Model file for the job. Use its own axes, mm. A direction names the side the tool comes from. Round coordinates to 2 decimals unless told otherwise and drop trailing zeros. Loops run counter-clockwise (first coordinate to the right, second up) from the corner with the lowest first, then second, coordinate; pieces in that order, holes last. Notation, with made-up numbers: (44.5, 82) - (58.5, 82) arc R32 ccw to (58.5, 118) - close; hole circle Ø1 at (-20, 22). An arc over 180 degrees is marked (long way). Use one line per item in the form item = value.
Autodesk Inventor part; units mm, degrees
ref_plane "YZ Plane" through (0, 0, 0) normal (1, 0, 0) x (0, 1, 0)
ref_plane "XZ Plane" through (0, 0, 0) normal (0, 1, 0) x (-1, 0, 0)
ref_plane "XY Plane" through (0, 0, 0) normal (0, 0, 1) x (1, 0, 0)
sketch "Boceto1" plane through (0, 0, 0) normal (0, 0, 1) x (1, 0, 0)
  line L0 (-10, 20) -> (10, 20)
  line L1 (10, 20) -> (10, -20)
  line L2 (10, -20) -> (-10, -20)
  line L3 (-10, -20) -> (-10, 20)
  line L4 (-10, 20) -> (10, -20) construction
  line L5 (6.3055, 0) -> (10, 0) construction
  line L6 (0, -12.611) -> (0, -20) construction
  line L7 (-8, 18) -> (8, 18)
  line L8 (8, 18) -> (8, -18)
  line L9 (8, -18) -> (-8, -18)
  line L10 (-8, -18) -> (-8, 18)
  line L11 (-8, 0) -> (-10, 0)
  line L12 (0, 18) -> (0, 20)
  point P0 (0, 0)
  point P1 (0, 0)
  dimension "d0" = 40
  dimension "d4" = 20
  dimension "d5" = 2
  dimension "d6" = 2
extrude "Extrusión1" add sketch "Boceto1" along normal blind 156 contours L0 L12 L7 L10 L11 L3 | L0 L1 L2 L3 L11 L10 L9 L8 L7 L12
properties part number "C_358_40_2"
1. Cut at A-A, the plane y = -13.5. Give the cut face in (x, z), plus the area to 3 significant figures.
Geometry check:
outline = (-10, 0) - (-8, 0) - (-8, 156) - (-10, 156) - close; (8, 0) - (10, 0) - (10, 156) - (8, 156) - close
area = 624 mm^2
2. Cut at B-B, the plane x = -6. Give the cut face in (y, z), plus the area to 3 significant figures.
Geometry check:
outline = (-20, 0) - (-18, 0) - (-18, 156) - (-20, 156) - close; (18, 0) - (20, 0) - (20, 156) - (18, 156) - close
area = 624 mm^2
3. Tool access for faces 1 (the flat face through (-8.2, 1.6, 0)), 2 (the flat face through (0, -18, 77)): list every direction of +Z, -Z, +X, -X, +Y, -Y with a clear straight run to the whole face (end or side of a thin tool).
Geometry check:
face_1 = -Z, +X, -X, +Y, -Y
face_2 = +Z, -Z
4. Pull direction Y, two halves, no side cores. Call faces 3 (the flat face through (0, 18, 77)), 4 (the flat face through (-8.2, 1.6, 156)), 5 (the flat face through (8, 0, 77)), 6 (the flat face through (0, 20, 77)): +Y half, -Y half, draft (parallel to the pull), parting line (faces both ways), or undercut.
Geometry check:
face_3 = undercut
face_4 = draft
face_5 = undercut
face_6 = +Y half
5. Cut at C-C, the plane z = 123.5. Give the cut face in (x, y).
Geometry check:
outline = (-10, -20) - (10, -20) - (10, 20) - (-10, 20) - close; hole (-8, -18) - (8, -18) - (8, 18) - (-8, 18) - close
6. Wall check: probe 1 along X at (y, z) = (-2, 121.5); probe 2 along Y at (x, z) = (0.5, 66.5). Give the ranges that are in metal, low to high.
Geometry check:
probe_1 = -10 to -8, 8 to 10
probe_2 = -20 to -18, 18 to 20
